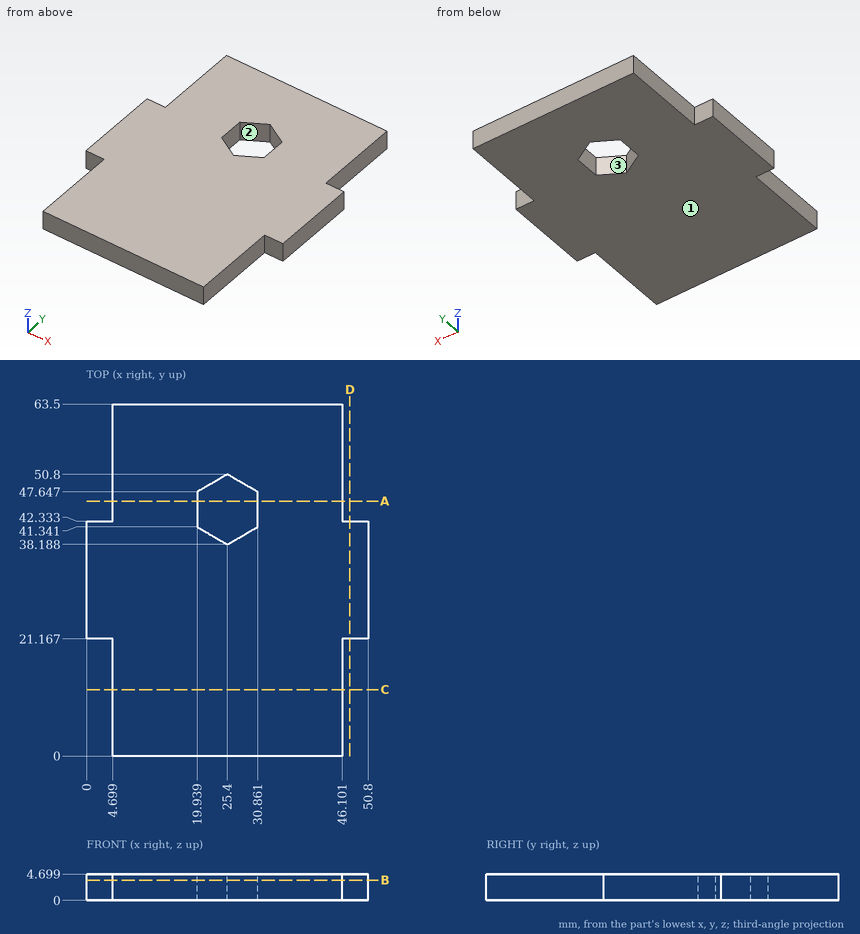
Could you check a few things on this drawing? It's one solid part, dimensions in mm from its lowest x, y, z. Coordinates: 2 decimals unless noted, no trailing zeros. Order: outer loops, then holes, each group sorted by start corner. A loop starts at its lowest first (then second) coordinate and runs counter-clockwise, first axis right, second up. Notation, with made-up numbers: (22, 58.5) - (55, 58.5) arc R31 cw to (55, 84.5) - close; hole circle Ø10 at (38, -40). An arc over 180 degrees is marked (long way). One line per question, with ' | ' between items.
(1) Suppose I cut it at A-A on y = 46. List the corners of the cut face in (x, z) for me.
Report:
outline: (4.7, 0) - (19.94, 0) - (19.94, 4.7) - (4.7, 4.7) - close; (30.86, 0) - (46.1, 0) - (46.1, 4.7) - (30.86, 4.7) - close
(2) Will these pins go through, and if not, where does the flat tip stop? pin 1 (2.5 mm diameter, centred on y = 54.5, z = 1.5, fed in from -X); pin 2 (2.5 mm diameter, centred on x = 49.5, z = 2, fed in from +Y); pin 3 (2.5 mm diameter, centred on x = 49.5, z = 1.5, fed in from -Y).
Report:
pin 1: stops at x = 4.7 | pin 2: stops at y = 42.33 | pin 3: stops at y = 21.17
(3) If we mould it in two halves opening along X, with no side actions, what happens to the marked faces 1, 2 and 3? For each: pulls with the +X half, pulls with the -X half, needs draft (parallel to the pull), parting line crosses it, or undercut.
Report:
face 1: needs draft | face 2: undercut | face 3: undercut
(4) Suppose I cut it at C-C on y = 12. List the corners of the cut face in (x, z) for me.
Report:
outline: (4.7, 0) - (46.1, 0) - (46.1, 4.7) - (4.7, 4.7) - close
(5) Suppose I cut it at D-D on x = 47.5. List the corners of the cut face in (y, z) for me.
Report:
outline: (21.17, 0) - (42.33, 0) - (42.33, 4.7) - (21.17, 4.7) - close
(6) Suppose I cut it at B-B on z = 3.65. List the corners of the cut face in (x, y) for me.
Report:
outline: (0, 21.17) - (4.7, 21.17) - (4.7, 0) - (46.1, 0) - (46.1, 21.17) - (50.8, 21.17) - (50.8, 42.33) - (46.1, 42.33) - (46.1, 63.5) - (4.7, 63.5) - (4.7, 42.33) - (0, 42.33) - close; hole (19.94, 41.34) - (25.4, 38.19) - (30.86, 41.34) - (30.86, 47.65) - (25.4, 50.8) - (19.94, 47.65) - close
(7) If I drill on L1, parallel to Y at x = 22, z = 1.2; L2, parallel to X at y = 14.5, z = 2.25; L3, parallel to X at y = 50, z = 1.8 (1 decimal), over which ranges is the centre line in solid material (lowest first)?
Report:
L1: y = 0 to 40.15, 48.84 to 63.5 | L2: x = 4.7 to 46.1 | L3: x = 4.7 to 24, 26.8 to 46.1
